```python
from build123d import *

# Parameters (mm, degrees)
SKETCH1_W           = 15
SKETCH1_H           = 85
BOSS_EXTRUDE1_DEPTH = 4
SKETCH2_W           = 12
SKETCH2_H           = 3
BOSS_EXTRUDE2_DEPTH = 10
CUT_EXTRUDE1_DEPTH  = 60
SKETCH4_R           = 1.6
CUT_EXTRUDE2_DEPTH  = 4
SKETCH5_W           = 10
SKETCH5_H           = 4
BOSS_EXTRUDE3_DEPTH = 50
SKETCH8_W           = 10
SKETCH8_H           = 40
CUT_EXTRUDE3_DEPTH  = 4
SKETCH10_W          = 10
SKETCH10_H          = 10
BOSS_EXTRUDE4_DEPTH = 40
SKETCH11_W          = 7
SKETCH11_H          = 10
BOSS_EXTRUDE5_DEPTH = 15
SKETCH13_W          = 5
SKETCH13_H          = 33
CUT_EXTRUDE4_DEPTH  = 10
CUT_EXTRUDE6_DEPTH  = 7
SKETCH17_W          = 4
SKETCH17_H          = 35
SKETCH17_H_2        = 40
BOSS_EXTRUDE6_DEPTH = 2
SKETCH18_W          = 4
SKETCH18_H          = 35
SKETCH18_H_2        = 40
BOSS_EXTRUDE7_DEPTH = 2
FILLET2_R           = 3
SKETCH19_W          = 4
SKETCH19_H          = 2.4
CUT_EXTRUDE7_DEPTH  = 10


with BuildPart() as part:
    # Sketch1 → Boss-Extrude1 (new body)
    with BuildSketch(Plane.XY):
        Rectangle(SKETCH1_W, SKETCH1_H)
    extrude(amount=BOSS_EXTRUDE1_DEPTH)

    # Sketch2 → Boss-Extrude2 (add)
    with BuildSketch(Plane.XY.offset(4)):
        with Locations((0, 27.5)):
            Rectangle(SKETCH2_W, SKETCH2_H)
        with Locations((0, -27.5)):
            Rectangle(SKETCH2_W, SKETCH2_H)
    extrude(amount=BOSS_EXTRUDE2_DEPTH)

    # Sketch3 → Cut-Extrude1 (cut)
    with BuildSketch(Plane(origin=(0, 29, 0), x_dir=(1, 0, 0), z_dir=(0, 1, 0))):
        with BuildLine():
            Line((0, -7.82217465), (0, -14))
            Line((0, -14), (4.896029025, -14))
            Line((4.896029025, -14), (0.904649293, -8.293404311))
            ThreePointArc((0.904649293, -8.293404311), (0.5100117, -7.947044007), (0, -7.82217465))
        make_face()
        with BuildLine():
            Line((-4.896029025, -14), (0, -14))
            Line((0, -14), (0, -7.82217465))
            ThreePointArc((0, -7.82217465), (-0.5100117, -7.947044007), (-0.904649293, -8.293404311))
            Line((-0.904649293, -8.293404311), (-4.896029025, -14))
        make_face()
    extrude(amount=-CUT_EXTRUDE1_DEPTH, mode=Mode.SUBTRACT)

    # Sketch4 → Cut-Extrude2 (cut)
    with BuildSketch(Plane.XY.offset(4)):
        with Locations((0, -15.4)):
            Circle(SKETCH4_R)
        Circle(SKETCH4_R)
    extrude(amount=-CUT_EXTRUDE2_DEPTH, mode=Mode.SUBTRACT)

    # Sketch5 → Boss-Extrude3 (add)
    with BuildSketch(Plane(origin=(0, 42.5, 0), x_dir=(1, 0, 0), z_dir=(0, 1, 0))):
        with Locations((12.5, -2)):
            Rectangle(SKETCH5_W, SKETCH5_H)
        with Locations((-12.5, -2)):
            Rectangle(SKETCH5_W, SKETCH5_H)
    extrude(amount=-BOSS_EXTRUDE3_DEPTH)

    # Sketch8 → Cut-Extrude3 (cut)
    with BuildSketch(Plane.XY.offset(4)):
        with Locations((12.5, 22.5)):
            Rectangle(SKETCH8_W, SKETCH8_H)
        with Locations((-12.5, 22.5)):
            Rectangle(SKETCH8_W, SKETCH8_H)
    extrude(amount=-CUT_EXTRUDE3_DEPTH, mode=Mode.SUBTRACT)

    # Sketch10 → Boss-Extrude4 (add)
    with BuildSketch(Plane.XY.offset(4)):
        with Locations((12.5, -2.5)):
            Rectangle(SKETCH10_W, SKETCH10_H)
        with Locations((-12.5, -2.5)):
            Rectangle(SKETCH10_W, SKETCH10_H)
    extrude(amount=BOSS_EXTRUDE4_DEPTH)

    # Sketch11 → Boss-Extrude5 (add)
    with BuildSketch(Plane.ZY.offset(-7.5)):
        with Locations((40.5, -2.5)):
            Rectangle(SKETCH11_W, SKETCH11_H)
    extrude(amount=BOSS_EXTRUDE5_DEPTH)

    # Sketch13 → Cut-Extrude4 (cut)
    with BuildSketch(Plane(origin=(0, 2.5, 0), x_dir=(1, 0, 0), z_dir=(0, 1, 0))):
        with Locations((-10, -20.5)):
            Rectangle(SKETCH13_W, SKETCH13_H)
        with Locations((10, -20.5)):
            Rectangle(SKETCH13_W, SKETCH13_H)
    extrude(amount=-CUT_EXTRUDE4_DEPTH, mode=Mode.SUBTRACT)

    # Sketch14 → Cut-Extrude6 (cut)
    with BuildSketch(Plane.XY.offset(44)):
        with BuildLine():
            ThreePointArc((0, 0.1), (-2.6, -2.5), (0, -5.1))
            Line((0, -5.1), (0, 0.1))
        make_face()
        with BuildLine():
            Line((0, 0.1), (0, -5.1))
            ThreePointArc((0, -5.1), (1.838477631, -4.338477631), (2.6, -2.5))
            ThreePointArc((2.6, -2.5), (1.838477631, -0.661522369), (0, 0.1))
        make_face()
    extrude(amount=-CUT_EXTRUDE6_DEPTH, mode=Mode.SUBTRACT)

    # Sketch17 → Boss-Extrude6 (add)
    with BuildSketch(Plane(origin=(7.5, 0, 0), x_dir=(0, 0, -1), z_dir=(1, 0, 0))):
        with Locations((-2, -25)):
            Rectangle(SKETCH17_W, SKETCH17_H)
        with Locations((-2, 22.5)):
            Rectangle(SKETCH17_W, SKETCH17_H_2)
    extrude(amount=BOSS_EXTRUDE6_DEPTH)

    # Sketch18 → Boss-Extrude7 (add)
    with BuildSketch(Plane.ZY.offset(7.5)):
        with Locations((2, -25)):
            Rectangle(SKETCH18_W, SKETCH18_H)
        with Locations((2, 22.5)):
            Rectangle(SKETCH18_W, SKETCH18_H_2)
    extrude(amount=BOSS_EXTRUDE7_DEPTH)

    # Fillet2
    fillet2_edges = [part.edges().sort_by_distance(p)[0] for p in [
        (9.5, -42.5, 2),
        (-9.5, -42.5, 2),
        (9.5, 42.5, 2),
        (-9.5, 42.5, 2),
        (-17.5, -2.5, 0),
        (17.5, -2.5, 44),
        (17.5, -2.5, 0),
        (-17.5, -2.5, 44),
        (12.5, -2.5, 37),
        (-12.5, -2.5, 37),
        (12.5, -2.5, 4),
        (-12.5, -2.5, 4),
    ]]
    fillet(fillet2_edges, radius=FILLET2_R)

    # Sketch19 → Cut-Extrude7 (cut)
    with BuildSketch(Plane(origin=(0, 2.5, 0), x_dir=(1, 0, 0), z_dir=(0, 1, 0))):
        with Locations((-2, -40.5)):
            Rectangle(SKETCH19_W, SKETCH19_H)
        with Locations((2, -40.5)):
            Rectangle(SKETCH19_W, SKETCH19_H)
    extrude(amount=-CUT_EXTRUDE7_DEPTH, mode=Mode.SUBTRACT)


solid = part.part
```
Can you work these out from the model? Positions are in its coordinate system, mm. A direction names the side the tool comes from. Coordinates: 2 decimals unless noted, no trailing zeros. Order: outer loops, then holes, each group sorted by start corner. A loop starts at its lowest first (then second) coordinate and runs counter-clockwise, first axis right, second up.
1. If we section it at B-B (y = -15.4): Please give me the cut outline in (x, z).
2. I need wall thicknesses on line 1 (Y direction, x = 0, z = 1); line 2 (Z direction, x = -1, y = -23); line 3 (Y direction, x = 14.5, z = 41). Which ranges of each line are inside material? Lowest first, please.
3. I'm going to push flat-ended pins straight in: pin 1 (4 mm diameter, centred on y = 30, z = 10, fed in from +X); pin 2 (3 mm diameter, centred on x = 0, y = 0, fed in from -Z); pin 3 (2 mm diameter, centred on y = -31, z = 3, fed in from +X). Where does each tip first touch, or does it pass through?
4. If we section it at A-A (z = 21): Please give me the cut outline in (x, y).
5. If we section it at D-D (y = 14.5): Please give me the cut outline in (x, z), then the cut area to 3 significant figures.
6. For faces 4 (the face through (11.6, -2.57, 4.86)), 5 (the face through (-1.27, -0.97, 2.03)), 6 (the face through (0, 26, 7)), which set-ups out of +Z, -Z, +X, -X, +Y, -Y let a thin tool reach every point of the face, with its end or its side?
7. Thinking about a two-plate mould opening in X: for faces 1 (the face through (-3, -1, 0)), 2 (the face through (-6, -28, 9)), 3 (the face through (2, -5, 37)), which applies, +X half, -X half, draft (parallel to the pull), parting line (faces both ways), or undercut?
8. If we section it at C-C (x = 13.5): Please give me the cut outline in (y, z), then the cut area to 3 significant figures.
Entries:
1. outline: (-9.5, 0) - (-1.6, 0) - (-1.6, 4) - (-9.5, 4) - close; (1.6, 0) - (9.5, 0) - (9.5, 4) - (1.6, 4) - close
2. line 1: y = -42.5 to -17, -13.8 to -1.6, 1.6 to 42.5
2. line 2: z = 0 to 4
2. line 3: y = -7.5 to 2.5
3. pin 1: stops at x = 6
3. pin 2: stops at z = 37
3. pin 3: stops at x = 9.5
4. outline: (-17.5, -7.5) - (-12.5, -7.5) - (-12.5, 2.5) - (-17.5, 2.5) - close; (12.5, -7.5) - (17.5, -7.5) - (17.5, 2.5) - (12.5, 2.5) - close
5. outline: (-9.5, 0) - (9.5, 0) - (9.5, 4) - (-9.5, 4) - close
5. area: 76.0 mm2
6. face 4: +Y, -Y
6. face 5: -Z
6. face 6: +Z, +X, -X
7. face 1: draft
7. face 2: -X half
7. face 3: undercut
8. outline: (-7.5, 0) - (2.5, 0) - (2.5, 44) - (-7.5, 44) - close
8. area: 440 mm2
